The listing builds one solid part. Answer for the finished solid, in the listing's coordinates (mm). Face numbers are marked on the shaded views. A direction names the side the tool comes from. Round coordinates to 2 decimals unless told otherwise and drop trailing zeros. Write each loop counter-clockwise with the first axis right and the second up, starting at its lowest first coordinate (ties: lowest second). Pieces come first, ordered by that corner, then holes.
Item 1: Find section B-B on x = 40.5. Give the vertices of the cut face in (y, z).
Item 2: For a pull along Z with two mould halves and no side action, classify the marked faces 3, 4 and 5 as +Z half, -Z half, draft (parallel to the pull), parting line (faces both ways), or undercut.
Item 3: Find section A-A on y = -19. Give the vertices of the cut face in (x, z).
Item 4: Each of these flat-tipped pins is pushed along its axis until it touches: pin 1 (19 mm diameter, centred on x = 23.5, y = -15.5, fed in from +Z); pin 2 (4 mm diameter, centred on y = -18, z = 20.5, fed in from -X); pin 3 (1 mm diameter, centred on y = -30, z = 10.5, fed in from +X). Where does it stop, or does it pass through?
Item 5: A tool of negligible diameter and unlimited length cuts with its end or side. For the marked faces 1 and 2, from which of +Z, -Z, +X, -X, +Y, -Y can it reach the whole face along a straight path? Write none if from no direction.
Item 6: Find section C-C on z = 3.5. Give the vertices of the cut face in (x, y).
Item 7: Find the intervals of material crossed by probe 1 along Z at (x, y) = (39, -15.5); probe 2 along X at (y, z) = (-20, 35.5); probe 3 along X at (y, z) = (-7, 27), in increasing order.
```python
from build123d import *

# Parameters (mm, degrees)
F1_DEPTH = 40
F3_DEPTH = 53


with BuildPart() as f1:
    # F0 (on Front) → F1 (new body)
    with BuildSketch(Plane.XZ):
        Polygon((10.352762, 38.637033), (0, 0), (50, 0), align=None)
    extrude(amount=F1_DEPTH)

    # F2 (on face) → F3 (cut)
    with BuildSketch(Plane.XZ.offset(40)):
        Polygon((44.86927, 5), (14.457346, 34.637033), (6.516127, 5), align=None)
    extrude(amount=-F3_DEPTH, mode=Mode.SUBTRACT)


solid = f1.part
```
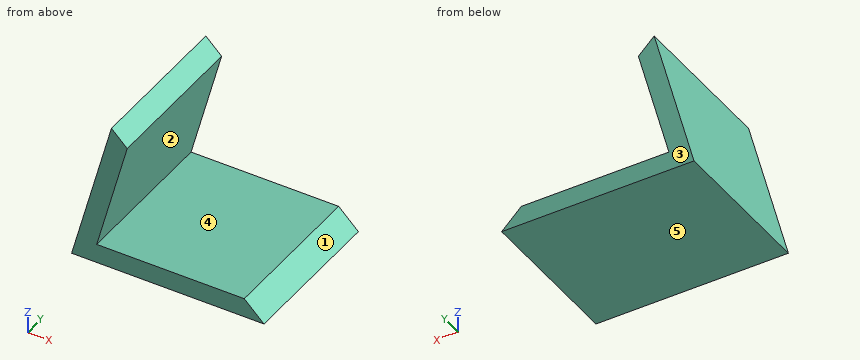
Check values:
1. outline: (-40, 0) - (0, 0) - (0, 5) - (-40, 5) - close
2. face 3: draft
2. face 4: undercut
2. face 5: -Z half
3. outline: (0, 0) - (50, 0) - (44.87, 5) - (6.52, 5) - (14.46, 34.64) - (10.35, 38.64) - close
4. pin 1: stops at z = 35.08
4. pin 2: stops at x = 4.96
4. pin 3: stops at x = 8.12
5. face 1: +Z, +X, +Y, -Y
5. face 2: +X, +Y, -Y
6. outline: (0.94, -40) - (46.41, -40) - (46.41, 0) - (0.94, 0) - close
7. probe 1: z = 0 to 5
7. probe 2: x = 9.51 to 13.57
7. probe 3: x = 7.23 to 12.41
